```python
from build123d import *

# Parameters (mm, degrees)
SWEEP1_PROFILE_R = 5
FILLET1_R        = 1


with BuildPart() as part:
    # Sweep1: sweep along a path in Sketch1
    with BuildLine(Plane.XY) as sweep1_path:
        Line((70, 0), (10, 0))
        ThreePointArc((10, 0), (2.928932188, 2.928932188), (0, 10))
        Line((0, 10), (0, 80))
    # Sweep1 profile (on start of the path) → Sweep1 (sweep)
    with BuildSketch(Plane(origin=(70, 0, 0), x_dir=(0, 0, -1), z_dir=(-1, 0, 0))):
        Circle(SWEEP1_PROFILE_R)
    sweep(path=sweep1_path.line)

    # Fillet1
    fillet1_edges = [part.edges().sort_by_distance(p)[0] for p in [
        (0, 80, 5),
        (70, 0, 5),
    ]]
    fillet(fillet1_edges, radius=FILLET1_R)


solid = part.part
```
Verification items for the finished model (mm, model axes). A direction names the side the tool comes from. Round coordinates to 2 decimals unless told otherwise and drop trailing zeros. Write each loop counter-clockwise with the first axis right and the second up, starting at its lowest first coordinate (ties: lowest second). Pieces come first, ordered by that corner, then holes. Notation, with made-up numbers: (17, 28) - (67, 28) arc R20 ccw to (67, 53) - close; hole circle Ø9 at (18, 44.5). An arc over 180 degrees is marked (long way). Answer as a JSON object with one key per item and string values. Group by question number.
Q1. Thickness scan on line 1 (Y direction, x = 47, z = -3); line 2 (Y direction, x = 14.5, z = 0); line 3 (X direction, y = 8, z = 2). Record the ranges inside material, lowest first.
Q2. Section check B-B, the plane y = 11. Enter the section's corners in (x, z), plus the area to 3 significant figures.
Q3. Tool access check on faces 1 (the cylindrical face through (39.09, 4.88, 1.08)), 2 (the cylindrical face through (4.88, 44.98, 1.08)), 3 (the flat face through (70, 0, 0)). Record the directions out of +Z, -Z, +X, -X, +Y, -Y that give a thin tool (end or side, any length) a straight path to the whole face; none if there is none.
Q4. Go/stop test with flat-tipped pins: pin 1 Ø1 at (y, z) = (28.5, 2.5) entering from +X; pin 2 Ø3 at (x, z) = (20, -3.5) entering from -Y; pin 3 Ø10 at (x, y) = (28.5, 12) entering from +Z; pin 4 Ø8 at (x, y) = (6, 48.5) entering from -Z. Record where each tip stops, or that it passes through.
Q5. Section check A-A, the plane z = 0. Enter the section's corners in (x, y).
Found:
{
 "1": {"line 1": "y = -4 to 4", "line 2": "y = -5 to 5", "line 3": "x = -4.44 to 4.97"},
 "2": {"outline": "circle Ø10 at (0, 0)", "area": "78.5 mm^2"},
 "3": {"face 1": "+X", "face 2": "+Y", "face 3": "+Z, -Z, +X, +Y, -Y"},
 "4": {"pin 1": "stops at x = 4.58", "pin 2": "stops at y = -4.58", "pin 3": "passes through", "pin 4": "stops at z = -4.58"},
 "5": {"outline": "(-5, 10) arc R15 ccw to (10, -5) - (69, -5) arc R1 ccw to (70, -4) - (70, 4) arc R1 ccw to (69, 5) - (10, 5) arc R5 cw to (5, 10) - (5, 79) arc R1 ccw to (4, 80) - (-4, 80) arc R1 ccw to (-5, 79) - close"}
}
